Part print with two shaded views. Sizes in mm from the minimum x, y, z corner. A direction names the side the tool comes from. Round coordinates to 2 decimals unless told otherwise and drop trailing zeros. Write each loop counter-clockwise with the first axis right and the second up, starting at its lowest first coordinate (ties: lowest second). Pieces come first, ordered by that corner, then holes. Notation, with made-up numbers: (-20.5, 48.25) -> (-5.5, 48.25) arc R20 ccw to (-5.5, 81.25) -> close; hole circle Ø3 at (-8.75, 7). An arc over 180 degrees is marked (long way). Answer in a Markdown table with one row per item.
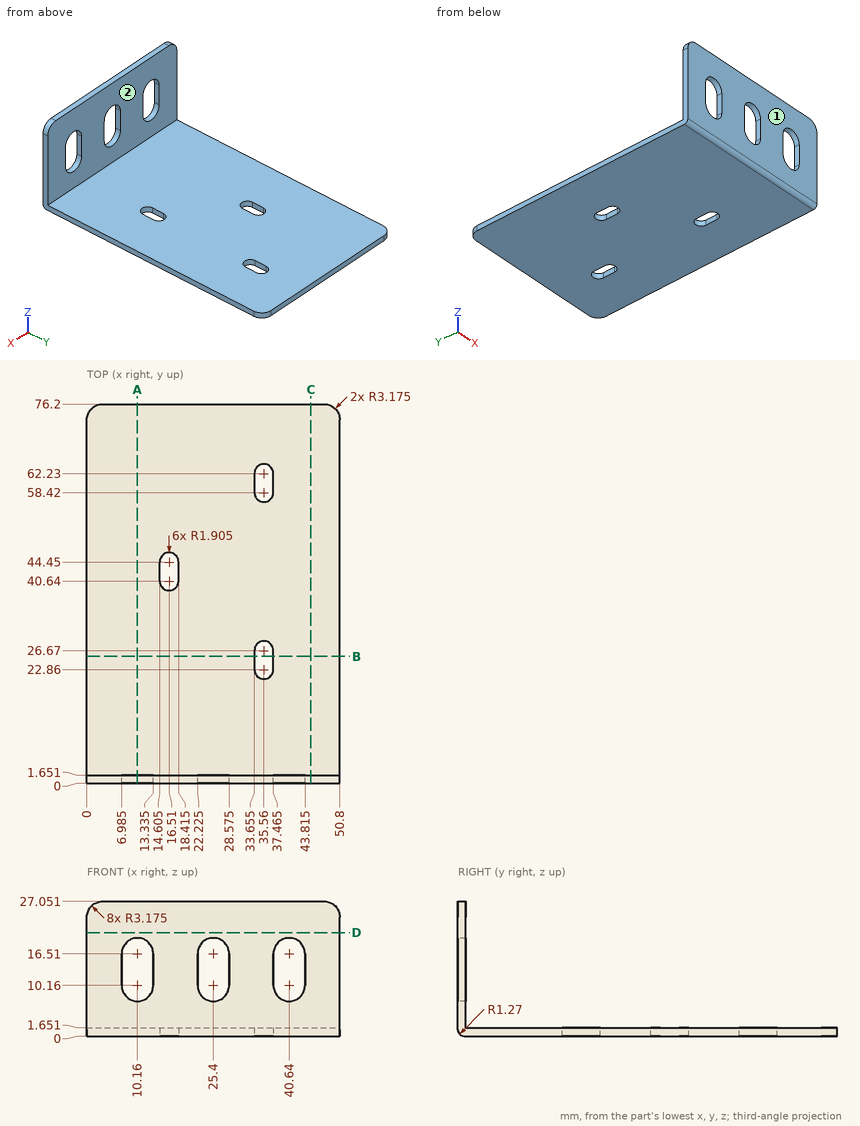
Q1. Wall check: line 1 (Z direction, x = 39.5, y = 37). Give the ranges that are in metal, low to high. Write a range as [from, to].
A:
| item | result |
|---|---|
| line 1 | [0, 1.65] |
Q2. Saw through at D-D on z = 20.75. Write the cut outline in (x, y), plus the area to 3 significant figures.
A:
| item | result |
|---|---|
| outline | (0, 0) -> (50.8, 0) -> (50.8, 1.65) -> (0, 1.65) -> close |
| area | 83.9 mm² |
Q3. Drop flat-ended pins along their axis: P1, Ø5, axis at x = 31.5, z = 20, coming from the +Y side; P2, Ø1, axis at x = 40, y = 53.5, coming from the +Z side. Give the stop position or say it passes through.
A:
| item | result |
|---|---|
| P1 | y = 1.65 |
| P2 | z = 1.65 |
Q4. Saw through at C-C on x = 45. Write the cut outline in (y, z).
A:
| item | result |
|---|---|
| outline | (0, 1.27) arc R1.27 ccw to (1.27, 0) -> (76.2, 0) -> (76.2, 1.65) -> (1.65, 1.65) -> (1.65, 27.05) -> (0, 27.05) -> close |
Q5. Saw through at A-A on x = 10.16. Write the cut outline in (y, z) (3 decimals).
A:
| item | result |
|---|---|
| outline | (0, 1.27) arc R1.27 ccw to (1.27, 0) -> (76.2, 0) -> (76.2, 1.651) -> (1.651, 1.651) -> (1.651, 6.985) -> (0, 6.985) -> close; (0, 19.685) -> (1.651, 19.685) -> (1.651, 27.051) -> (0, 27.051) -> close |
Q6. Saw through at B-B on y = 25.5. Write the cut outline in (x, z) (3 decimals).
A:
| item | result |
|---|---|
| outline | (0, 0) -> (33.655, 0) -> (33.655, 1.651) -> (0, 1.651) -> close; (37.465, 0) -> (50.8, 0) -> (50.8, 1.651) -> (37.465, 1.651) -> close |
Q7. Which spindle directions (+Z, -Z, +X, -X, +Y, -Y) get a long thin tool onto all of the face, cutting with end or side? Do the marked faces 1 and 2. Say none if no direction does.
A:
| item | result |
|---|---|
| face 1 | +Z, -Z, +X, -X, -Y |
| face 2 | +Z, +X, -X, +Y |
